```python
from build123d import *

# Parameters (mm, degrees)
CUT_EXTRUDE1_START = -5.08
CUT_EXTRUDE1_DEPTH = 5.08
SKETCH2_W          = 17.78
SKETCH2_H          = 57.15
CUT_EXTRUDE2_DEPTH = 77.379704765
SKETCH3_W          = 17.78
SKETCH3_H          = 57.15
CUT_EXTRUDE3_DEPTH = 77.379704765
SKETCH4_W          = 17.78
SKETCH4_H          = 57.15
CUT_EXTRUDE4_DEPTH = 77.379704765
CUT_EXTRUDE5_DEPTH = 77.379704765
CUT_EXTRUDE6_DEPTH = 77.379704765
CUT_EXTRUDE7_DEPTH = 77.379704765
CUT_EXTRUDE8_DEPTH = 77.379704765
FILLET1_R          = 3.175
SKETCH11_R         = 1.8
CUT_EXTRUDE9_DEPTH = 77.379704765


with BuildPart() as part:
    # Cut-Extrude1: read off the stored shape, not the designer's step
    # Cut-Extrude1 outline → Cut-Extrude1 (new body)
    with BuildSketch(Plane.XZ.offset(CUT_EXTRUDE1_START)):
        Polygon((-12.7, -12.7), (-12.7, -69.85), (30.48, -69.85), (30.48, 69.85), (-30.48, 69.85), (-30.48, -12.7), align=None)
    extrude(amount=CUT_EXTRUDE1_DEPTH)

    # Sketch2 → Cut-Extrude2 (cut, through all)
    with BuildSketch(Plane.XZ):
        with Locations((-21.59, 41.275)):
            Rectangle(SKETCH2_W, SKETCH2_H)
    extrude(amount=-CUT_EXTRUDE2_DEPTH, mode=Mode.SUBTRACT)

    # Sketch3 → Cut-Extrude3 (cut, through all)
    with BuildSketch(Plane.XZ):
        with Locations((21.59, 41.275)):
            Rectangle(SKETCH3_W, SKETCH3_H)
    extrude(amount=-CUT_EXTRUDE3_DEPTH, mode=Mode.SUBTRACT)

    # Sketch4 → Cut-Extrude4 (cut, through all)
    with BuildSketch(Plane.XZ):
        with Locations((21.59, -41.275)):
            Rectangle(SKETCH4_W, SKETCH4_H)
    extrude(amount=-CUT_EXTRUDE4_DEPTH, mode=Mode.SUBTRACT)

    # Sketch5 → Cut-Extrude5 (cut, through all)
    with BuildSketch(Plane(origin=(0, 5.08, 0), x_dir=(-1, 0, 0), z_dir=(0, 1, 0))):
        with BuildLine():
            Line((2.413, -62.357), (2.413, -11.938))
            ThreePointArc((2.413, -11.938), (0, -9.525), (-2.413, -11.938))
            Line((-2.413, -11.938), (-2.413, -62.357))
            ThreePointArc((-2.413, -62.357), (0, -64.77), (2.413, -62.357))
        make_face()
    extrude(amount=-CUT_EXTRUDE5_DEPTH, mode=Mode.SUBTRACT)

    # Sketch6 → Cut-Extrude6 (cut, through all)
    with BuildSketch(Plane(origin=(0, 5.08, 0), x_dir=(-1, 0, 0), z_dir=(0, 1, 0))):
        with BuildLine():
            Line((-2.413, 62.357), (-2.413, 11.938))
            ThreePointArc((-2.413, 11.938), (0, 9.525), (2.413, 11.938))
            Line((2.413, 11.938), (2.413, 62.357))
            ThreePointArc((2.413, 62.357), (0, 64.77), (-2.413, 62.357))
        make_face()
    extrude(amount=-CUT_EXTRUDE6_DEPTH, mode=Mode.SUBTRACT)

    # Sketch7 → Cut-Extrude7 (cut, through all)
    with BuildSketch(Plane(origin=(0, 5.08, 0), x_dir=(-1, 0, 0), z_dir=(0, 1, 0))):
        with BuildLine():
            Line((-23.495, -2.413), (-11.43, -2.413))
            ThreePointArc((-11.43, -2.413), (-9.017, 0), (-11.43, 2.413))
            Line((-11.43, 2.413), (-23.495, 2.413))
            ThreePointArc((-23.495, 2.413), (-25.908, 0), (-23.495, -2.413))
        make_face()
    extrude(amount=-CUT_EXTRUDE7_DEPTH, mode=Mode.SUBTRACT)

    # Sketch8 → Cut-Extrude8 (cut, through all)
    with BuildSketch(Plane.XZ):
        with BuildLine():
            Line((-23.495, -2.413), (-11.43, -2.413))
            ThreePointArc((-11.43, -2.413), (-9.017, 0), (-11.43, 2.413))
            Line((-11.43, 2.413), (-23.495, 2.413))
            ThreePointArc((-23.495, 2.413), (-25.908, 0), (-23.495, -2.413))
        make_face()
    extrude(amount=-CUT_EXTRUDE8_DEPTH, mode=Mode.SUBTRACT)

    # Fillet1
    fillet1_edges = [part.edges().sort_by_distance(p)[0] for p in [
        (-30.48, 2.54, -12.7),
        (-12.7, 2.54, -12.7),
        (-12.7, 2.54, -69.85),
        (-12.7, 2.54, 69.85),
        (-12.7, 2.54, 12.7),
        (-30.48, 2.54, 12.7),
        (12.7, 2.54, 69.85),
        (30.48, 2.54, 12.7),
        (12.7, 2.54, 12.7),
        (30.48, 2.54, -12.7),
        (12.7, 2.54, -69.85),
        (12.7, 2.54, -12.7),
    ]]
    fillet(fillet1_edges, radius=FILLET1_R)

    # Sketch11 → Cut-Extrude9 (cut, through all)
    with BuildSketch(Plane(origin=(0, 5.08, 0), x_dir=(1, 0, 0), z_dir=(0, 1, 0))):
        with Locations(Location((0, 0, 0), (0, 0, 270))):
            Circle(SKETCH11_R)
    extrude(amount=-CUT_EXTRUDE9_DEPTH, mode=Mode.SUBTRACT)


solid = part.part
```
Source: CAD feature listing. Evaluate the final solid. Frame: model axes, mm. A direction names the side the tool comes from. Give positions to 0.01 mm unless a question says otherwise; leave off trailing zeros. Order: outer loops, then holes, each group sorted by start corner. A loop starts at its lowest first (then second) coordinate and runs counter-clockwise, first axis right, second up.
(1) Contact query for flat-ended pins moving along their axis: P1, Ø2.5, axis at x = 17.5, y = 3.5, coming from the -Z side; P2, Ø1.5, axis at x = 18.5, y = 3, coming from the +Z side; P3, Ø1.5, axis at y = 1.5, z = 43, coming from the -X side. Output: stop coordinate, or through.
(2) Material intervals for line 1 along X through (y, z) = (3.65, 0); line 2 along X through (y, z) = (1.3, -25), sorted ascending.
(3) Section query D-D (z = 55). Return the cut outline in (x, y).
(4) Access query for faces 1 (the face through (-13.65, 2.58, 13.61)), 2 (the face through (22, 3, -12.7)), 3 (the face through (22, 3, 12.7)), 4 (the face through (-2.413, 3, 37)), 5 (the face through (-2, 0, 0)). Directions: +Z, -Z, +X, -X, +Y, -Y. A direction counts if a zero-diameter tool reaches every point of the face in a straight line with its end or side. Return the directions, or none.
(5) Section query C-C (x = -22). Return the cut outline in (y, z).
(6) Section query B-B (x = 0). Return the cut outline in (y, z) (3 decimals), plus the area to 3 significant figures.
(7) Pull-direction query (Z, two-part tool) for faces 6 (the face through (2.413, 3, -37)), 7 (the face through (29.53, 2.58, 11.79)), 8 (the face through (-13.61, 2.5, -13.65)); classes: +Z half, -Z half, draft (parallel to the pull), parting line (faces both ways), or undercut.
(8) Section query A-A (z = 0). Return the cut outline in (x, y), plus the area to 3 significant figures.
Outcome:
1. P1: stops at z = -12.7
1. P2: stops at z = 12.7
1. P3: stops at x = -12.7
2. line 1: x = -30.48 to -25.91, -9.02 to -1.8, 1.8 to 9.02, 25.91 to 30.48
2. line 2: x = -12.7 to -2.41, 2.41 to 12.7
3. outline: (-12.7, 0) - (-2.41, 0) - (-2.41, 5.08) - (-12.7, 5.08) - close; (2.41, 0) - (12.7, 0) - (12.7, 5.08) - (2.41, 5.08) - close
4. face 1: +Z, -X, +Y, -Y
4. face 2: -Z, +X, +Y, -Y
4. face 3: +Z, +X, +Y, -Y
4. face 4: +Y, -Y
4. face 5: +Z, -Z, +X, -X, -Y
5. outline: (0, -12.7) - (5.08, -12.7) - (5.08, -2.41) - (0, -2.41) - close; (0, 2.41) - (5.08, 2.41) - (5.08, 12.7) - (0, 12.7) - close
6. outline: (0, -69.85) - (5.08, -69.85) - (5.08, -64.77) - (0, -64.77) - close; (0, -9.525) - (5.08, -9.525) - (5.08, -1.8) - (0, -1.8) - close; (0, 1.8) - (5.08, 1.8) - (5.08, 9.525) - (0, 9.525) - close; (0, 64.77) - (5.08, 64.77) - (5.08, 69.85) - (0, 69.85) - close
6. area: 130 mm2
7. face 6: undercut
7. face 7: +Z half
7. face 8: -Z half
8. outline: (-30.48, 0) - (-25.91, 0) - (-25.91, 5.08) - (-30.48, 5.08) - close; (-9.02, 0) - (-1.8, 0) - (-1.8, 5.08) - (-9.02, 5.08) - close; (1.8, 0) - (9.02, 0) - (9.02, 5.08) - (1.8, 5.08) - close; (25.91, 0) - (30.48, 0) - (30.48, 5.08) - (25.91, 5.08) - close
8. area: 120 mm2
